Design review of the part built by this model. Coordinates are the model's own, in mm. Face numbers are marked on the shaded views. Coordinates: 2 decimals unless noted, no trailing zeros. Order: outer loops, then holes, each group sorted by start corner. A loop starts at its lowest first (then second) coordinate and runs counter-clockwise, first axis right, second up. Notation, with made-up numbers: (20, 7) -> (44, 7) arc R29 cw to (44, 31) -> close; hole circle Ø7 at (-21, 65). An arc over 180 degrees is marked (long way). Use a Markdown table: item, result. Add a question column.
Q1. Add section B-B (y = -40.5). State the section outline as (x, z) points, then the cut area to 3 significant figures.
Q2. Add section A-A (y = 75). State the section outline as (x, z) points.
Q3. Insertion check: pin 1 (5 mm diameter, centred on y = 49.5, z = 0, fed in from -X); pin 2 (4.5 mm diameter, centred on x = 53.26, y = -30.75, fed in from -Z); pin 3 (8 mm diameter, centred on y = -28.5, z = 0, fed in from -X); pin 4 (1.8 mm diameter, centred on y = 83.5, z = 10, fed in from -X). Each pin has a flat end and moves straight along its axis. Give the tip position at first contact, or say it passes through.
Q4. Add section C-C (y = 28). State the section outline as (x, z) points.
Q5. The part is to be moulded in two halves that separate along X. For the marked faces 1, 2 and 3, say which applies: pulls with the +X half, pulls with the -X half, needs draft (parallel to the pull), parting line crosses it, or undercut.
Q6. Wall thickness on probe 1 along Y at (x, z) = (0, 3.75); probe 2 along Y at (x, z) = (0, -3); probe 3 along Z at (x, y) = (32, 56): over which ranges is each line inside the solid? List them lowest first.
from build123d import *

# Parameters (mm, degrees)
BOSS_EXTRUDE1_DEPTH      = 5.5
BOSS_EXTRUDE1_DEPTH_BACK = 5.5
SKETCH1_R                = 68
SKETCH1_R_2              = 49
SKETCH2_W                = 43
SKETCH2_H                = 43
SKETCH2_R                = 18.5
BOSS_EXTRUDE2_DEPTH      = 11
SKETCH3_R                = 1.7
CUT_EXTRUDE1_DEPTH       = 138.932048488
SKETCH4_R                = 2.95
CUT_EXTRUDE2_DEPTH       = 3
CUT_EXTRUDE3_START       = -5.5
SKETCH5_W                = 67
SKETCH5_H                = 21
SKETCH5_R                = 1.7
CUT_EXTRUDE3_DEPTH       = 5.5
SKETCH6_R                = 1.7
CUT_EXTRUDE4_DEPTH       = 138.932048488
SKETCH7_R                = 1.7
CUT_EXTRUDE5_DEPTH       = 138.932048488
CIRPATTERN1_COUNT        = 3
CUT_EXTRUDE6_DEPTH       = 3
CIRPATTERN2_COUNT        = 3
SKETCH10_R               = 2.95
CUT_EXTRUDE8_DEPTH       = 3
CIRPATTERN4_COUNT        = 3
BOSS_EXTRUDE4_DEPTH      = 9.5
SKETCH14_W               = 41.4
SKETCH14_H               = 7
CUT_EXTRUDE10_DEPTH      = 178.251234128
FILLET2_R                = 1


with BuildPart() as part:
    # Sketch1 → Boss-Extrude1 (new, two sides: drawn at the far end of the back side and taken through both)
    with BuildSketch(Plane.XY.offset(-BOSS_EXTRUDE1_DEPTH_BACK)):
        Circle(SKETCH1_R)
        Circle(SKETCH1_R_2, mode=Mode.SUBTRACT)
    extrude(amount=BOSS_EXTRUDE1_DEPTH + BOSS_EXTRUDE1_DEPTH_BACK)

    # Sketch2 → Boss-Extrude2 (add)
    # profile 1 of 7: a face of its own
    with BuildSketch(Plane(origin=(0, 0, -5.5), x_dir=(-1, 0, 0), z_dir=(0, 0, -1))):
        with BuildLine():
            Line((-33.5, 66.5), (-33.5, 93.149074069))
            ThreePointArc((-33.5, 93.149074069), (-38.168927278, 67.100269686), (-51.594405594, 44.294664592))
            ThreePointArc((-51.594405594, 44.294664592), (-34.722076366, 58.466891596), (-14.203872711, 66.5))
            Line((-14.203872711, 66.5), (-33.5, 66.5))
        make_face()
    # profile 2 of 7: a face of its own
    with BuildSketch(Plane(origin=(0, 0, -5.5), x_dir=(-1, 0, 0), z_dir=(0, 0, -1))):
        with BuildLine():
            ThreePointArc((-14.203872711, 66.5), (-34.722076366, 58.466891596), (-51.594405594, 44.294664592))
            Line((-51.594405594, 44.294664592), (-20.951913723, 44.294664592))
            ThreePointArc((-20.951913723, 44.294664592), (0, 49), (20.951913723, 44.294664592))
            Line((20.951913723, 44.294664592), (51.594405594, 44.294664592))
            ThreePointArc((51.594405594, 44.294664592), (34.722076366, 58.466891596), (14.203872711, 66.5))
            Line((14.203872711, 66.5), (-14.203872711, 66.5))
        make_face()
    # profile 3 of 7: a face of its own
    with BuildSketch(Plane(origin=(0, 0, -5.5), x_dir=(-1, 0, 0), z_dir=(0, 0, -1))):
        with BuildLine():
            ThreePointArc((51.594405594, 44.294664592), (38.168927278, 67.100269686), (33.5, 93.149074069))
            Line((33.5, 93.149074069), (33.5, 66.5))
            Line((33.5, 66.5), (14.203872711, 66.5))
            ThreePointArc((14.203872711, 66.5), (34.722076366, 58.466891596), (51.594405594, 44.294664592))
        make_face()
    # profile 4 of 7: a face of its own
    with BuildSketch(Plane(origin=(0, 0, -5.5), x_dir=(-1, 0, 0), z_dir=(0, 0, -1))):
        with BuildLine():
            ThreePointArc((14.203872711, 66.5), (0, 68), (-14.203872711, 66.5))
            Line((-14.203872711, 66.5), (14.203872711, 66.5))
        make_face()
    # profile 5 of 7: a face of its own
    with BuildSketch(Plane(origin=(0, 0, -5.5), x_dir=(-1, 0, 0), z_dir=(0, 0, -1))):
        with BuildLine():
            Line((-21.5, 76.5), (-21.5, 119.5))
            Line((-21.5, 119.5), (-33.5, 119.5))
            Line((-33.5, 119.5), (-33.5, 93.149074069))
            Line((-33.5, 93.149074069), (-33.5, 66.5))
            Line((-33.5, 66.5), (-14.203872711, 66.5))
            ThreePointArc((-14.203872711, 66.5), (0, 68), (14.203872711, 66.5))
            Line((14.203872711, 66.5), (33.5, 66.5))
            Line((33.5, 66.5), (33.5, 93.149074069))
            Line((33.5, 93.149074069), (33.5, 119.5))
            Line((33.5, 119.5), (21.5, 119.5))
            Line((21.5, 119.5), (21.5, 76.5))
            Line((21.5, 76.5), (-21.5, 76.5))
        make_face()
    # profile 6 of 7: a face of its own
    with BuildSketch(Plane(origin=(0, 0, -5.5), x_dir=(-1, 0, 0), z_dir=(0, 0, -1))):
        with Locations((0, 98)):
            Rectangle(SKETCH2_W, SKETCH2_H)
        with Locations((0, 98)):
            Circle(SKETCH2_R, mode=Mode.SUBTRACT)
    # profile 7 of 7: a face of its own
    with BuildSketch(Plane(origin=(0, 0, -5.5), x_dir=(-1, 0, 0), z_dir=(0, 0, -1))):
        with Locations((0, 98)):
            Circle(SKETCH2_R)
    extrude(amount=-BOSS_EXTRUDE2_DEPTH)

    # Sketch3 → Cut-Extrude1 (cut, through all)
    with BuildSketch(Plane.XY.offset(5.5)):
        with Locations((-21.5, 113.5)):
            Circle(SKETCH3_R)
        with Locations((-21.5, 102.5)):
            Circle(SKETCH3_R)
        with Locations(Location((21.5, 113.5, 0), (0, 0, 180))):
            Circle(SKETCH3_R)
        with Locations(Location((21.5, 102.5, 0), (0, 0, 180))):
            Circle(SKETCH3_R)
    extrude(amount=-CUT_EXTRUDE1_DEPTH, mode=Mode.SUBTRACT)

    # Sketch4 → Cut-Extrude2 (cut)
    with BuildSketch(Plane.XY.offset(5.5)):
        with Locations((-21.5, 113.5)):
            Circle(SKETCH4_R)
        with Locations((-21.5, 102.5)):
            Circle(SKETCH4_R)
        with Locations((21.5, 102.5)):
            Circle(SKETCH4_R)
        with Locations((21.5, 113.5)):
            Circle(SKETCH4_R)
    extrude(amount=-CUT_EXTRUDE2_DEPTH, mode=Mode.SUBTRACT)

    # Sketch5 → Cut-Extrude3 (cut)
    # profile 1 of 2: a face of its own
    with BuildSketch(Plane(origin=(0, 0, -5.5), x_dir=(-1, 0, 0), z_dir=(0, 0, -1)).offset(CUT_EXTRUDE3_START)):
        with Locations((0, 109)):
            Rectangle(SKETCH5_W, SKETCH5_H)
        with Locations(Location((-21.5, 102.5, 0), (0, 0, 180))):
            Circle(SKETCH5_R, mode=Mode.SUBTRACT)
        with Locations(Location((-21.5, 113.5, 0), (0, 0, 180))):
            Circle(SKETCH5_R, mode=Mode.SUBTRACT)
        with Locations(Location((21.5, 102.5, 0), (0, 0, 180))):
            Circle(SKETCH5_R, mode=Mode.SUBTRACT)
        with Locations(Location((21.5, 113.5, 0), (0, 0, 180))):
            Circle(SKETCH5_R, mode=Mode.SUBTRACT)
    # profile 2 of 2: a face of its own
    with BuildSketch(Plane(origin=(0, 0, -5.5), x_dir=(-1, 0, 0), z_dir=(0, 0, -1)).offset(CUT_EXTRUDE3_START)):
        with BuildLine():
            Line((33.5, 98.5), (-33.5, 98.5))
            ThreePointArc((-33.5, 98.5), (0, 85.618054906), (33.5, 98.5))
        make_face()
    extrude(amount=CUT_EXTRUDE3_DEPTH, mode=Mode.SUBTRACT)

    # Sketch6 → Cut-Extrude4 (cut, through all)
    with BuildSketch(Plane(origin=(0, 0, -5.5), x_dir=(-1, 0, 0), z_dir=(0, 0, -1))):
        with Locations((0, 61.5)):
            Circle(SKETCH6_R)
        with Locations((53.260562333, -30.75)):
            Circle(SKETCH6_R)
        with Locations((-53.260562333, -30.75)):
            Circle(SKETCH6_R)
    extrude(amount=-CUT_EXTRUDE4_DEPTH, mode=Mode.SUBTRACT)

    # Sketch7 → Cut-Extrude5 (cut, through all)
    with BuildSketch(Plane(origin=(0, 0, -5.5), x_dir=(-1, 0, 0), z_dir=(0, 0, -1))):
        with Locations((0, 53)):
            Circle(SKETCH7_R)
    cut_extrude5 = extrude(amount=-CUT_EXTRUDE5_DEPTH, mode=Mode.SUBTRACT)

    # CirPattern1: Cut-Extrude5 ×3 about axis
    cirpattern1_axis = Axis((0, 0, 0), (0, 0, 1))
    for i in range(1, CIRPATTERN1_COUNT):
        add(cut_extrude5.rotate(cirpattern1_axis, i * 360 / CIRPATTERN1_COUNT), mode=Mode.SUBTRACT)

    # Sketch8 → Cut-Extrude6 (cut)
    with BuildSketch(Plane.XY.offset(2.5)):
        Polygon((-3.35, 47.346917497), (3.35, 47.346917497), (3.35, 53), (1.675, 50.098814897), (-1.675, 50.098814897), (-3.35, 53), align=None)
        Polygon((-3.35, 53), (-1.675, 55.901185103), (1.675, 55.901185103), (3.35, 53), (1.675, 50.098814897), (-1.675, 50.098814897), align=None)
    cut_extrude6 = extrude(amount=-CUT_EXTRUDE6_DEPTH, mode=Mode.SUBTRACT)

    # CirPattern2: Cut-Extrude6 ×3 about axis
    cirpattern2_axis = Axis((0, 0, 0), (0, 0, 1))
    for i in range(1, CIRPATTERN2_COUNT):
        add(cut_extrude6.rotate(cirpattern2_axis, i * 360 / CIRPATTERN2_COUNT), mode=Mode.SUBTRACT)

    # Sketch10 → Cut-Extrude8 (cut)
    with BuildSketch(Plane.XY.offset(5.5)):
        with Locations((0, 61.5)):
            Circle(SKETCH10_R)
    cut_extrude8 = extrude(amount=-CUT_EXTRUDE8_DEPTH, mode=Mode.SUBTRACT)

    # CirPattern4: Cut-Extrude8 ×3 about axis
    cirpattern4_axis = Axis((0, 0, 0), (0, 0, 1))
    for i in range(1, CIRPATTERN4_COUNT):
        add(cut_extrude8.rotate(cirpattern4_axis, i * 360 / CIRPATTERN4_COUNT), mode=Mode.SUBTRACT)

    # Sketch13 → Boss-Extrude4 (add)
    with BuildSketch(Plane.XY.offset(5.5)):
        with BuildLine():
            Line((-23.7, 95), (-23.7, 60.525283973))
            ThreePointArc((-23.7, 60.525283973), (0, 65), (23.7, 60.525283973))
            Line((23.7, 60.525283973), (23.7, 95))
            Line((23.7, 95), (-23.7, 95))
        make_face()
    extrude(amount=BOSS_EXTRUDE4_DEPTH)

    # Sketch14 → Cut-Extrude10 (cut, through all)
    with BuildSketch(Plane(origin=(0, 95, 0), x_dir=(1, 0, 0), z_dir=(0, 1, 0))):
        with Locations((0, -9)):
            Rectangle(SKETCH14_W, SKETCH14_H)
    extrude(amount=-CUT_EXTRUDE10_DEPTH, mode=Mode.SUBTRACT)

    # Fillet2
    fillet2_edges = [part.edges().sort_by_distance(p)[0] for p in [
        (0, 65, 15),
        (-23.7, 60.525283973, 10.25),
        (23.7, 77.762641986, 15),
        (23.7, 60.525283973, 10.25),
        (0, 95, 15),
        (23.7, 95, 10.25),
        (-23.7, 77.762641986, 15),
        (-23.7, 95, 10.25),
        (22.206695396, 61.08897347, 5.5),
        (-23.7, 77.762641986, 5.5),
        (-22.2, 95, 5.5),
        (23.7, 77.762641986, 5.5),
        (22.2, 95, 5.5),
        (-22.206695396, 61.08897347, 5.5),
        (-20.7, 61.615825889, 9),
        (20.7, 61.615825889, 9),
        (0, 65, 12.5),
        (-20.7, 78.307912945, 5.5),
        (20.7, 78.307912945, 5.5),
        (-20.7, 95, 9),
        (0, 95, 12.5),
        (20.7, 95, 9),
    ]]
    fillet(fillet2_edges, radius=FILLET2_R)


solid = part.part
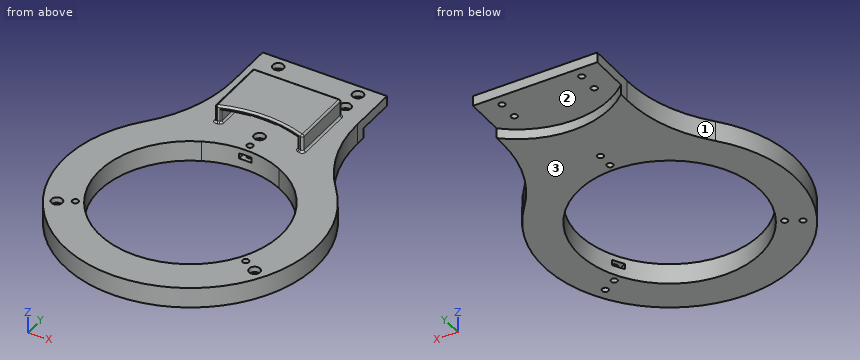
Established:
| question | item | result |
|---|---|---|
| 1 | outline | (-54.62, -5.5) -> (-27.58, -5.5) -> (-27.58, 5.5) -> (-54.62, 5.5) -> close; (27.58, -5.5) -> (54.62, -5.5) -> (54.62, 5.5) -> (27.58, 5.5) -> close |
| 1 | area | 595 mm^2 |
| 2 | outline | (-35.73, -5.5) -> (35.73, -5.5) -> (35.73, 5.5) -> (24.7, 5.5) arc R1 cw to (23.7, 6.5) -> (23.7, 14) arc R1 ccw to (22.7, 15) -> (-22.7, 15) arc R1 ccw to (-23.7, 14) -> (-23.7, 6.5) arc R1 cw to (-24.7, 5.5) -> (-35.73, 5.5) -> close; hole (-20.7, 6.5) arc R1 ccw to (-19.7, 5.5) -> (19.7, 5.5) arc R1 ccw to (20.7, 6.5) -> (20.7, 12.5) -> (-20.7, 12.5) -> close |
| 3 | pin 1 | x = -49.38 |
| 3 | pin 2 | z = -5.5 |
| 3 | pin 3 | x = -63.43 |
| 3 | pin 4 | x = -23.7 |
| 4 | outline | (-61.97, -5.5) -> (-40.21, -5.5) -> (-40.21, 5.5) -> (-61.97, 5.5) -> close; (40.21, -5.5) -> (61.97, -5.5) -> (61.97, 5.5) -> (40.21, 5.5) -> close |
| 5 | face 1 | pulls with the -X half |
| 5 | face 2 | undercut |
| 5 | face 3 | needs draft |
| 6 | probe 1 | -68 to -49, 49 to 51.3, 54.7 to 58.55, 64.45 to 119.5 |
| 6 | probe 2 | -68 to -49, 49 to 51.3, 54.7 to 59.8, 63.2 to 85.62 |
| 6 | probe 3 | -5.5 to 5.5 |
